For this review, take the finished solid that the model builds, in its own axes (mm). A direction names the side the tool comes from. Give positions to 0.01 mm unless a question says otherwise; leave off trailing zeros. Write each loop counter-clockwise with the first axis right and the second up, starting at its lowest first coordinate (ties: lowest second). Pieces come first, ordered by that corner, then holes.
from build123d import *

# Parameters (mm, degrees)
F0_R           = 8
F1_DEPTH       = 13
F2_DEPTH       = 20
F4_D           = 9
F4_CBORE_D     = 15
F4_CBORE_DEPTH = 10
F5_R           = 1
F6_SIZE2       = 1
F6_SIZE        = 1


with BuildPart() as f1:
    # F0 (on Top) → F1 (new body)
    with BuildSketch(Plane.XY):
        with BuildLine():
            Line((43, 50), (43, 0))
            Line((43, 0), (66.5621155816, 13.7777614045))
            ThreePointArc((66.5621155816, 13.7777614045), (73, 25), (66.5621155816, 36.2222385955))
            Line((66.5621155816, 36.2222385955), (43, 50))
        make_face()
        with Locations((60, 25)):
            Circle(F0_R, mode=Mode.SUBTRACT)
    extrude(amount=F1_DEPTH)

    # F0 (on Top) → F2 (join)
    with BuildSketch(Plane.XY):
        with BuildLine():
            Line((0, 24.5), (0, 0))
            Line((0, 0), (43, 0))
            Line((43, 0), (43, 50))
            Line((43, 50), (0, 50))
            Line((0, 50), (0, 25.5))
            Line((0, 25.5), (19.5, 25.5))
            Line((19.5, 25.5), (19.5, 31.7823299831))
            ThreePointArc((19.5, 31.7823299831), (30, 37.5), (40.5, 31.7823299831))
            Line((40.5, 31.7823299831), (40.5, 18.2176700169))
            ThreePointArc((40.5, 18.2176700169), (30, 12.5), (19.5, 18.2176700169))
            Line((19.5, 18.2176700169), (19.5, 24.5))
            Line((19.5, 24.5), (0, 24.5))
        make_face()
    extrude(amount=F2_DEPTH)

    # F4 (through all)
    with Locations(Plane(origin=(0, 50, 0), x_dir=(-1, 0, 0), z_dir=(0, 1, 0))):
        with Locations((-10, 10)):
            CounterBoreHole(F4_D / 2, F4_CBORE_D / 2, F4_CBORE_DEPTH)

    # F5
    f5_edges = [f1.edges().sort_by_distance(p)[0] for p in [
        (0, 0, 10),
        (21.5, 50, 20),
        (0, 37.75, 20),
        (21.5, 0, 20),
        (43, 25, 20),
        (30, 37.5, 20),
        (30, 12.5, 20),
        (40.5, 25, 20),
        (19.5, 21.358835, 20),
        (19.5, 28.641165, 20),
        (0, 25.5, 10),
        (54.781058, 6.888881, 13),
        (0, 12.25, 20),
        (0, 24.5, 10),
        (0, 50, 10),
        (54.781058, 43.111119, 13),
        (73, 25, 13),
    ]]
    fillet(f5_edges, radius=F5_R)

    # F6
    f6_edges = [f1.edges().sort_by_distance(p)[0] for p in [
        (52, 25, 13),
        (17.5, 50, 10),
    ]]
    chamfer(f6_edges, length=F6_SIZE, length2=F6_SIZE2)


solid = f1.part
(1) The part is to be moulded in two halves that separate along Z. For faces 1 (the flat face through (10, 25.5, 5)), 2 (the flat face through (10, 40, 5)), 3 (the flat face through (36, 36.5, 0)), 4 (the cylindrical face through (54.8, 7.23, 12.7)), say which applies: +Z half, -Z half, draft (parallel to the pull), parting line (faces both ways), or undercut.
(2) We need section A-A (x = 10). Write out the cut boundary in (y, z).
(3) For L1, parallel to Z at x = 16, y = 42.5; L2, parallel to X at y = 28, z = 1.5; L3, parallel to Y at x = 4, z = 7.25, list the stretches that pass through material, from the lowest coordinate up.
(4) Tool access review of faces 5 (the flat face through (0, 12, 9)), 6 (the cylindrical face through (30.2, 12.5, 9.4)), 7 (the flat face through (10, 24.5, 5)): name each direction out of +Z, -Z, +X, -X, +Y, -Y from which nothing blocks a thin tool from reaching the whole face with its end or side.
(5) We need section B-B (z = 10). Count the separate pieces of the cut face and the enclosed holes in it, and give its area (3 significant figures).
(6) Clearance check with flat-ended pins moving along their axes: pin 1 Ø2 at (x, z) = (8, 6) entering from +Y; pin 2 Ø5.5 at (y, z) = (24.5, 15.5) entering from +X; pin 3 Ø8 at (y, z) = (44.5, 6.5) entering from +X. State where each tip first meets the part, or that it passes through.
The answers:
1. face 1: draft
1. face 2: undercut
1. face 3: -Z half
1. face 4: +Z half
2. outline: (0, 0) - (24.5, 0) - (24.5, 5.5) - (0, 5.5) - close; (0, 14.5) - (24.5, 14.5) - (24.5, 20) - (1, 20) arc R1 ccw to (0, 19) - close; (25.5, 0) - (50, 0) - (50, 1.5) - (49, 2.5) - (40, 2.5) - (40, 5.5) - (25.5, 5.5) - close; (25.5, 14.5) - (40, 14.5) - (40, 17.5) - (49, 17.5) - (50, 18.5) - (50, 19) arc R1 ccw to (49, 20) - (25.5, 20) - close
3. L1: z = 0 to 5.5, 14.5 to 20
3. L2: x = 0 to 19.5, 40.5 to 52.58, 67.42 to 72.65
3. L3: y = 0 to 24.5, 25.5 to 40
4. face 5: +Z, -Z, -X, +Y, -Y
4. face 6: +Z, -Z
4. face 7: +Z, -Z, -X
5. separate pieces: 3
5. enclosed holes: 1
5. area: 1,930 mm2
6. pin 1: stops at y = 40
6. pin 2: stops at x = 72.65
6. pin 3: stops at x = 59.25
